The listing builds one solid part. Answer for the finished solid, in the listing's coordinates (mm). A direction names the side the tool comes from. Give positions to 0.01 mm unless a question says otherwise; leave off trailing zeros. Write each loop counter-clockwise with the first axis right and the second up, starting at its lowest first coordinate (ties: lowest second). Pieces come first, ordered by that corner, then holes. Notation, with made-up numbers: (60, 53) -> (117, 53) arc R18 ccw to (117, 65) -> close; hole circle Ø10 at (81, 3). An arc over 180 degrees is marked (long way). Put each result on its own line as item: value. Start each with the question number.
1) A cutting plane is placed at B-B (x = -17). Write down the section's boundary in (y, z), then the cut area to 3 significant figures.
2) Find the intervals of material crossed by line 1 along Z through (x, y) = (-5.25, 18.5); line 2 along Y through (x, z) = (-1.5, 16); line 3 along Y through (x, z) = (7, 20), in increasing order. Write a range as from..to.
3) Flat-ended cylindrical pins translate along their axes: pin 1 Ø5 at (y, z) = (-47, 11.5) entering from +X; pin 2 Ø12 at (x, y) = (-4, -104) entering from +Z; pin 3 Ø2.5 at (x, y) = (0.5, -44) entering from +Z; pin 4 Ø7.5 at (y, z) = (19.5, 32) entering from +X. Find the tip coordinate at first contact, or state that the pin passes through.
4) For faces 1 (the flat face through (2, -48, 4)), 2 (the flat face through (-12, -4.33, 22)), 3 (the flat face through (0, -116, 22.5)), determine the directions among +Z, -Z, +X, -X, +Y, -Y from which every point of the face is accessible in a straight line to the end or side of a thin tool.
5) For a pull along Z with two mould halves and no side action, classify faces 4 (the flat face through (0, -81.67, 6)), 5 (the flat face through (-12.52, 2.2, 18.77)), 6 (the flat face through (2, -109, 5)) as released by +Z, released by -Z, zero draft, split by the parting line, or undercut.
6) A cutting plane is placed at A-A (y = -111). Write down the section's boundary in (x, z), then the cut area to 4 significant figures.
7) A cutting plane is placed at D-D (z = 39.5). Write down the section's boundary in (x, y), then the cut area to 3 significant figures.
8) A cutting plane is placed at C-C (y = 18.5). Write down the section's boundary in (x, z).
Autodesk Fusion 360 part; units mm, degrees
sketch "Sketch3" plane through (0, 0, 0) normal (0, 0, 1) x (1, 0, 0)
  circle A0 centre (0, 0) radius 11
  line L0 (0, 11) -> (0, 26)
  line L1 (0, 26) -> (-20, 26)
  line L2 (-20, 26) -> (-20, -26)
  line L3 (-20, -26) -> (0, -26)
  line L4 (0, -26) -> (0, -11)
  line L5 (0, -26) -> (20, -26)
  line L6 (-20, -26) -> (-20, -106)
  line L7 (-20, -106) -> (20, -106)
  line L8 (20, -106) -> (20, -26)
  dimension "d15" = 22
  dimension "d16" = 15
  dimension "d17" = 20
  dimension "d18" = 52
  dimension "d19" = 20
  dimension "d20" = 80
  dimension "d21" = 40
extrude "Extrude4" add sketch "Sketch3" along normal blind 45 contours A0 L0 L1 L2 L3 L4
extrude "Extrude5" add sketch "Sketch3" along normal blind 22.5 contours L3 L5 L6 L7 L8
sketch "Sketch4" plane through (-20, 0, 0) normal (-1, 0, 0) x (0, -1, 0)
  line L0 (-26, 0) -> (106, 0)
  line L1 (106, 0) -> (106, 22.5)
  line L2 (106, 22.5) -> (26, 22.5)
  line L3 (26, 22.5) -> (26, 45)
  line L4 (26, 45) -> (-26, 45)
  line L5 (-26, 45) -> (-26, 0)
  line L6 (-26, 45) -> (-18.5, 45) construction
  line L7 (26, 45) -> (18.5, 45) construction
  line L8 (-18.5, 45) -> (-18.5, 33) construction
  circle A0 centre (-18.5, 33) radius 2.5
  circle A1 centre (18.5, 33) radius 2.5
  circle A2 centre (-18.5, 12) radius 2.5
  circle A3 centre (18.5, 12) radius 2.5
  line L9 (-26, 45) -> (26, 45) construction
  line L10 (0, 45) -> (0, 0) construction
  circle A4 centre (0, 22.5) radius 2.5
  dimension "d26" = 7.5
  dimension "d27" = 7.5
  dimension "d28" = 12
  dimension "d29" = 5
  dimension "d32" = 37
  dimension "d33" = -21
  dimension "d36" = 5
extrude "Extrude6" cut sketch "Sketch4" against normal blind 40 contours A0 | A1 | A2 | A3 | A4
sketch "Sketch5" plane through (-20, 0, 0) normal (-1, 0, 0) x (0, -1, 0)
  circle A0 centre (18.5, 33) radius 2.5
  circle A1 centre (18.5, 12) radius 2.5
  circle A2 centre (-18.5, 33) radius 2.5
  circle A3 centre (-18.5, 12) radius 2.5
  line L0 (-26, 0) -> (106, 0)
  line L1 (106, 0) -> (106, 22.5)
  line L2 (106, 22.5) -> (26, 22.5)
  line L3 (26, 22.5) -> (26, 45)
  line L4 (26, 45) -> (-26, 45)
  line L5 (-26, 45) -> (-26, 0)
  circle A4 centre (0, 22.5) radius 2.5
  circle A5 centre (-18.5, 33) radius 5
  circle A6 centre (18.5, 33) radius 5
  circle A7 centre (-18.5, 12) radius 5
  circle A8 centre (18.5, 12) radius 5
  dimension "d37" = 10
  dimension "d40" = 37
  dimension "d41" = -21
sketch "Sketch6" plane through (-20, 0, 0) normal (-1, 0, 0) x (0, -1, 0)
  line L0 (106, 22.5) -> (86, 22.5) construction
  circle A0 centre (86, 22.5) radius 15
  circle A1 centre (46, 22.5) radius 15
  dimension "d42" = 20
  dimension "d43" = 30
  dimension "d46" = -40
  dimension "d47" = 0
extrude "Extrude7" cut sketch "Sketch6" against normal blind 400
sketch "Sketch7" plane through (-20, 0, 0) normal (-1, 0, 0) x (0, -1, 0)
  line L0 (0, 22.5) -> (0, 27.5) construction
  line L1 (0, 27.5) -> (-4.3301, 25)
  line L2 (-4.3301, 25) -> (-4.3301, 20)
  line L3 (-4.3301, 20) -> (0, 17.5)
  line L4 (0, 17.5) -> (4.3301, 20)
  line L5 (4.3301, 20) -> (4.3301, 25)
  line L6 (4.3301, 25) -> (0, 27.5)
  point P0 (0, 22.5)
  dimension "d50" = 5
extrude "Extrude8" cut sketch "Sketch7" against normal blind 5 from surface at -6
sketch "Sketch8" plane through (0, 0, 0) normal (0, 0, -1) x (1, 0, 0)
  line L0 (0, -26) -> (0, -11)
  arc A0 (0, 11) -> (0, -11) centre (0, 0) ccw
  line L1 (0, 11) -> (0, 26)
  line L2 (0, 26) -> (20, 26)
  line L3 (20, 26) -> (20, 106)
  line L4 (20, 106) -> (-20, 106)
  line L5 (-20, 106) -> (-20, -26)
  line L6 (-20, -26) -> (0, -26)
  line L7 (0, 26) -> (0, 46) construction
  circle A1 centre (0, 46) radius 2.5
  circle A2 centre (0, 86) radius 2.5
  dimension "d54" = 20
  dimension "d55" = 5
  dimension "d58" = 0
  dimension "d59" = 40
extrude "Extrude9" cut sketch "Sketch8" against normal blind 20 contours A1 | A2
sketch "Sketch9" plane through (0, 0, 0) normal (0, 0, -1) x (1, 0, 0)
  circle A0 centre (0, 46) radius 2.5
  circle A1 centre (0, 86) radius 2.5
  line L0 (0, -26) -> (0, -11)
  arc A2 (0, 11) -> (0, -11) centre (0, 0) ccw
  line L1 (0, 11) -> (0, 26)
  line L2 (0, 26) -> (20, 26)
  line L3 (20, 26) -> (20, 106)
  line L4 (20, 106) -> (-20, 106)
  line L5 (-20, 106) -> (-20, -26)
  line L6 (-20, -26) -> (0, -26)
  line L7 (0, 46) -> (-5, 46) construction
  line L8 (0, 86) -> (-5, 86) construction
  line L9 (-5, 46) -> (-2.5, 41.6699)
  line L10 (-2.5, 41.6699) -> (2.5, 41.6699)
  line L11 (2.5, 41.6699) -> (5, 46)
  line L12 (5, 46) -> (2.5, 50.3301)
  line L13 (2.5, 50.3301) -> (-2.5, 50.3301)
  line L14 (-2.5, 50.3301) -> (-5, 46)
  line L15 (-5, 86) -> (-2.5, 81.6699)
  line L16 (-2.5, 81.6699) -> (2.5, 81.6699)
  line L17 (2.5, 81.6699) -> (5, 86)
  line L18 (5, 86) -> (2.5, 90.3301)
  line L19 (2.5, 90.3301) -> (-2.5, 90.3301)
  line L20 (-2.5, 90.3301) -> (-5, 86)
  point P0 (0, 46)
  point P1 (0, 86)
  dimension "d62" = 5
  dimension "d63" = 5
extrude "Extrude10" cut sketch "Sketch9" against normal blind 6 from surface at -4 contours L9 L10 L11 L12 L13 L14 | L15 L16 L17 L18 L19 L20
sketch "Sketch10" plane through (-20, 0, 0) normal (-1, 0, 0) x (0, -1, 0)
  arc A0 (71, 22.5) -> (101, 22.5) centre (86, 22.5) ccw
  line L0 (71, 22.5) -> (61, 22.5)
  arc A1 (31, 22.5) -> (61, 22.5) centre (46, 22.5) ccw
  line L1 (31, 22.5) -> (26, 22.5)
  line L2 (26, 22.5) -> (26, 45)
  line L3 (26, 45) -> (-26, 45)
  line L4 (-26, 45) -> (-26, 0)
  line L5 (-26, 0) -> (106, 0)
  line L6 (106, 0) -> (106, 22.5)
  line L7 (106, 22.5) -> (101, 22.5)
  circle A2 centre (0, 22.5) radius 2.5
  circle A3 centre (-18.5, 33) radius 2.5
  circle A4 centre (-18.5, 12) radius 2.5
  circle A5 centre (18.5, 33) radius 2.5
  circle A6 centre (18.5, 12) radius 2.5
  circle A7 centre (-18.5, 12) radius 5
  circle A8 centre (-18.5, 33) radius 5
  circle A9 centre (18.5, 33) radius 5
  circle A10 centre (18.5, 12) radius 5
  dimension "d67" = 10
  dimension "d68" = 10
  dimension "d69" = 10
  dimension "d70" = 10
extrude "Extrude11" cut sketch "Sketch10" against normal blind 5 contours A7 | A8 | A9 | A10
sketch "Sketch11" plane through (0, 0, 0) normal (0, 0, -1) x (1, 0, 0)
  circle A0 centre (0, 46) radius 2.5
  circle A1 centre (0, 86) radius 2.5
  line L0 (0, -26) -> (0, -11)
  arc A2 (0, 11) -> (0, -11) centre (0, 0) ccw
  line L1 (0, 11) -> (0, 26)
  line L2 (0, 26) -> (20, 26)
  line L3 (20, 26) -> (20, 106)
  line L4 (20, 106) -> (-20, 106)
  line L5 (-20, 106) -> (-20, -26)
  line L6 (-20, -26) -> (0, -26)
  line L7 (-20, 106) -> (20, 106)
  line L8 (20, 106) -> (20, 121)
  line L9 (20, 121) -> (-20, 121)
  line L10 (-20, 121) -> (-20, 106)
  dimension "d73" = 15
extrude "Extrude12" add sketch "Sketch11" against normal blind 22.5 contours L4 L7 L8 L9 L10
sketch "Sketch12" plane through (0, 0, 22.5) normal (0, 0, 1) x (-1, 0, 0)
  line L0 (-20, 101) -> (20, 101)
  line L1 (20, 101) -> (20, 121)
  line L2 (20, 121) -> (-20, 121)
  line L3 (-20, 121) -> (-20, 101)
  line L4 (0, 101) -> (0, 121) construction
  circle A0 centre (0, 111) radius 2.5
  dimension "d76" = 5
extrude "Extrude13" cut sketch "Sketch12" against normal blind 22.5 contours A0
sketch "Sketch13" plane through (0, 0, 0) normal (0, 0, -1) x (1, 0, 0)
  circle A0 centre (0, 111) radius 2.5
  circle A1 centre (0, 46) radius 2.5
  circle A2 centre (0, 86) radius 2.5
  line L0 (0, -26) -> (0, -11)
  arc A3 (0, 11) -> (0, -11) centre (0, 0) ccw
  line L1 (0, 11) -> (0, 26)
  line L2 (0, 26) -> (20, 26)
  line L3 (20, 26) -> (20, 121)
  line L4 (20, 121) -> (-20, 121)
  line L5 (-20, 121) -> (-20, -26)
  line L6 (-20, -26) -> (0, -26)
  circle A4 centre (0, 111) radius 5
  dimension "d79" = 10
extrude "Extrude14" cut sketch "Sketch13" against normal blind 5 contours A4
equation "d51 = 0 mm - 6.00 mm"
Reply:
1. outline: (-121, 0) -> (26, 0) -> (26, 45) -> (-26, 45) -> (-26, 22.5) -> (-31, 22.5) arc R15 cw to (-61, 22.5) -> (-71, 22.5) arc R15 cw to (-101, 22.5) -> (-121, 22.5) -> close; hole circle Ø10 at (-18.5, 12); hole circle Ø10 at (-18.5, 33); hole circle Ø5 at (0, 22.5); hole circle Ø10 at (18.5, 12); hole circle Ø10 at (18.5, 33)
1. area: 3,440 mm2
2. line 1: z = 0..9.5, 14.5..30.5, 35.5..45
2. line 2: y = -121..-113, -109..-99.52, -72.48..-59.52, -32.48..-10.9, 10.9..26
2. line 3: y = -121..-100.79, -71.21..-60.79, -31.21..-26
3. pin 1: passes through
3. pin 2: stops at z = 22.5
3. pin 3: stops at z = 4
3. pin 4: stops at x = 0
4. face 1: +Z
4. face 2: +X
4. face 3: +Z, +X, -X, -Y
5. face 4: zero draft
5. face 5: undercut
5. face 6: released by -Z
6. outline: (-20, 0) -> (-5, 0) -> (-5, 5) -> (-2.5, 5) -> (-2.5, 22.5) -> (-20, 22.5) -> close; (2.5, 5) -> (5, 5) -> (5, 0) -> (20, 0) -> (20, 22.5) -> (2.5, 22.5) -> close
6. area: 762.5 mm2
7. outline: (-20, -26) -> (0, -26) -> (0, -11) arc R11 cw to (0, 11) -> (0, 26) -> (-20, 26) -> close
7. area: 850 mm2
8. outline: (-20, 0) -> (0, 0) -> (0, 9.5) -> (-15, 9.5) -> (-15, 7) -> (-20, 7) -> close; (-20, 17) -> (-15, 17) -> (-15, 14.5) -> (0, 14.5) -> (0, 30.5) -> (-15, 30.5) -> (-15, 28) -> (-20, 28) -> close; (-20, 38) -> (-15, 38) -> (-15, 35.5) -> (0, 35.5) -> (0, 45) -> (-20, 45) -> close
